Geometry: final body of the model. Coordinates: model frame, mm. Face numbers are marked on the shaded views. A direction names the side the tool comes from. Coordinates: 2 decimals unless noted, no trailing zeros. Write each loop counter-clockwise with the first axis right and the second up, starting at its lowest first coordinate (ties: lowest second). Pieces come first, ordered by that corner, then holes. Notation, with made-up numbers: (83, 56.5) - (108, 56.5) arc R19 ccw to (108, 85.5) - close; hole circle Ø5 at (36.25, 46.25). An arc over 180 degrees is marked (long way). Answer as a JSON object with one key per item and string values. Group by question number.
Item 1: Section B-B on x = 44.5. Return loops of the section in (y, z), and give its area (3 significant figures).
Item 2: Set-up query: the marked faces 1, 2, 3 and 4. Return all of +Z, -Z, +X, -X, +Y, -Y with unobstructed straight access to the full face (end or side cutting, diameter ignored); none if empty.
Item 3: First-contact query: pin 1 Ø1.5 at (x, z) = (34.5, 3) entering from +Y; pin 2 Ø0.8 at (y, z) = (3, 4) entering from +X; pin 3 Ø5.5 at (x, z) = (52.5, 0) entering from +Y. Flat tips, straight axial feed; report the tip coordinate or a pass-through.
Item 4: Line query: line 1 along X through (y, z) = (-0.5, -4); line 2 along Z through (x, y) = (22, 0.25); line 3 along X through (y, z) = (-4.25, -2.5). Output: solid intervals per line, ascending. Write a range as from..to.
Item 5: Section C-C on y = 6.75. Return loops of the section in (x, z), and give its area (3 significant figures).
Item 6: Mould query, pull axis X, two halves, no side actions, for the marked faces 5, 6 and 7. Classes: pulls with the +X half, pulls with the -X half, needs draft (parallel to the pull), parting line crosses it, or undercut.
Item 7: Section D-D on x = 11.5. Return loops of the section in (y, z), and give its area (3 significant figures).
```python
from build123d import *

# Parameters (mm, degrees)
CHAMFER1_SIZE       = 1
BOSS_EXTRUDE1_START = -19
BOSS_EXTRUDE1_DEPTH = 19
CHAMFER2_SIZE       = 1
SKETCH3_OUTSIDE_W   = 26.814
SKETCH3_OUTSIDE_H   = 33.814
CUT_EXTRUDE1_DEPTH  = 20
SKETCH4_W           = 10
SKETCH4_H           = 4.464883459


with BuildPart() as part:
    # Sketch1 → Revolve1 (revolve)
    with BuildSketch(Plane.XY, mode=Mode.PRIVATE) as revolve1_sk:
        Polygon((0, 0), (0, 6), (20, 6), (20, 5), (60, 5), (60, 0), align=None)
    revolve(revolve1_sk.sketch.rotate(Axis((0, 0, 0), (1, 0, 0)), 90), axis=Axis((0, 0, 0), (1, 0, 0)))

    # Chamfer1
    chamfer1_edges = [part.edges().sort_by_distance(p)[0] for p in [
        (60, 0, -5),
        (20, 0, -6),
    ]]
    chamfer(chamfer1_edges, length=CHAMFER1_SIZE - 0.0001)  # a hair under: the kernel refuses the full size

    # Sketch2 → Boss-Extrude1 (add)
    with BuildSketch(Plane.ZY.offset(BOSS_EXTRUDE1_START)):
        with BuildLine():
            ThreePointArc((2.861817604, 10.9), (0, 13), (-2.861817604, 10.9))
            Line((-2.861817604, 10.9), (-5.723635209, 1.8))
            ThreePointArc((-5.723635209, 1.8), (0, 6), (5.723635209, 1.8))
            Line((5.723635209, 1.8), (2.861817604, 10.9))
        make_face()
    extrude(amount=BOSS_EXTRUDE1_DEPTH)

    # Chamfer2
    chamfer2_edges = [part.edges().sort_by_distance(p)[0] for p in [
        (0, -5.930506355, -0.910546196),
        (0, 6.35, 4.292726406),
        (0, 13, 0),
        (0, 6.35, -4.292726406),
    ]]
    chamfer(chamfer2_edges, length=CHAMFER2_SIZE)

    # Sketch3 outside → Cut-Extrude1 (cut)
    with BuildSketch(Plane(origin=(60, 0, 0), x_dir=(0, 0, -1), z_dir=(1, 0, 0))):
        with Locations((0, 3.5)):
            Rectangle(SKETCH3_OUTSIDE_W, SKETCH3_OUTSIDE_H)
        Polygon((5, 0), (2.5, 4.330127019), (-2.5, 4.330127019), (-5, 0), (-2.5, -4.330127019), (2.5, -4.330127019), align=None, mode=Mode.SUBTRACT)
    extrude(amount=-CUT_EXTRUDE1_DEPTH, mode=Mode.SUBTRACT)

    # Sketch4 → Cut-Revolve1 (revolve, cut)
    with BuildSketch(Plane.XY, mode=Mode.PRIVATE) as cut_revolve1_sk:
        with Locations((30, 5.732441729)):
            Rectangle(SKETCH4_W, SKETCH4_H)
    revolve(cut_revolve1_sk.sketch.rotate(Axis((40, 0, 0), (-1, 0, 0)), 270), axis=Axis((40, 0, 0), (-1, 0, 0)), mode=Mode.SUBTRACT)


solid = part.part
```
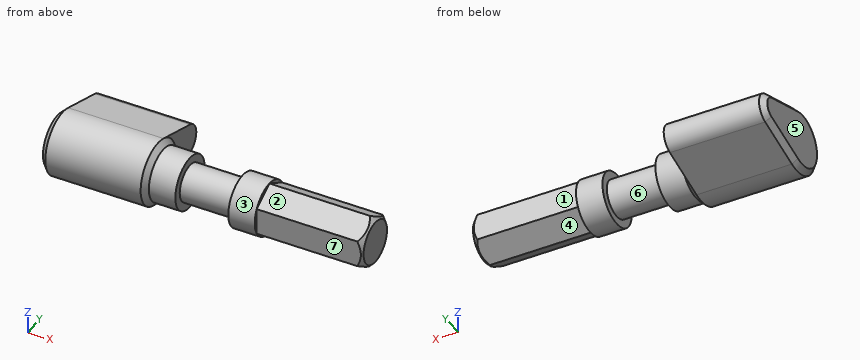
Checks:
{
 "1": {"outline": "(-4.33, -2.5) - (0, -5) - (4.33, -2.5) - (4.33, 2.5) - (0, 5) - (-4.33, 2.5) - close", "area": "65.0 mm^2"},
 "2": {"face 1": "+Z, -Z, +X, +Y", "face 2": "+Z, +X, -Y", "face 3": "+X", "face 4": "-Z, +X, +Y"},
 "3": {"pin 1": "y = 4.36", "pin 2": "x = 40", "pin 3": "y = 4.33"},
 "4": {"line 1": "0..25, 35..59.97", "line 2": "-4.99..4.99", "line 3": "0..25, 35..59.07"},
 "5": {"outline": "(0, -3.12) - (1, -4.17) - (19, -4.17) - (19, 4.17) - (1, 4.17) - (0, 3.12) - close", "area": "157 mm^2"},
 "6": {"face 5": "pulls with the -X half", "face 6": "undercut", "face 7": "needs draft"},
 "7": {"outline": "(1.8, -5.72) - (10.9, -2.86) arc R3 ccw to (10.9, 2.86) - (1.8, 5.72) arc R6 ccw (long way) to start", "area": "165 mm^2"}
}
